CAD build for the part. Positions are in the model's coordinates, mm. Face numbers are marked on the shaded views. Coordinates: 2 decimals unless noted, no trailing zeros. Loops run counter-clockwise (first coordinate to the right, second up) from the corner with the lowest first, then second, coordinate; pieces in that order, holes last. Notation, with made-up numbers: (28.5, 8) -> (55.5, 8) arc R18 cw to (55.5, 25) -> close; hole circle Ø1 at (23, 52). An arc over 180 degrees is marked (long way). Write each question's results on one line, items separated by ' | '.
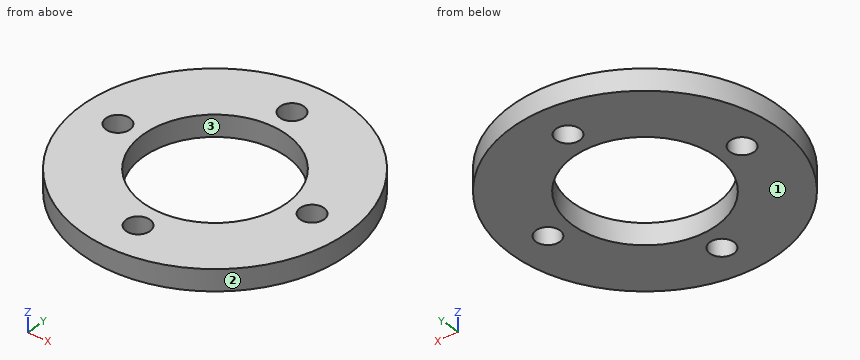
```python
from build123d import *

# Parameters (mm, degrees)
SKETCH1_R           = 25
SKETCH1_R_2         = 13.5
BOSS_EXTRUDE1_DEPTH = 4
SKETCH2_R           = 2.25
CUT_EXTRUDE1_DEPTH  = 5


with BuildPart() as part:
    # Sketch1 → Boss-Extrude1 (new body)
    with BuildSketch(Plane.XY):
        Circle(SKETCH1_R)
        Circle(SKETCH1_R_2, mode=Mode.SUBTRACT)
    extrude(amount=BOSS_EXTRUDE1_DEPTH)

    # Sketch2 → Cut-Extrude1 (cut, through all)
    with BuildSketch(Plane.XY.offset(4)):
        with Locations((0, 18)):
            Circle(SKETCH2_R)
        with Locations((18, 0)):
            Circle(SKETCH2_R)
        with Locations((0, -18)):
            Circle(SKETCH2_R)
        with Locations((-18, 0)):
            Circle(SKETCH2_R)
    extrude(amount=-CUT_EXTRUDE1_DEPTH, mode=Mode.SUBTRACT)


solid = part.part
```
Q1. Drop flat-ended pins along their axis: pin 1 (2 mm diameter, centred on x = -5.5, z = 2.5, fed in from -Y); pin 2 (4 mm diameter, centred on x = -18, y = 0, fed in from -Z); pin 3 (2 mm diameter, centred on y = 3.5, z = 2.5, fed in from +X); pin 4 (2 mm diameter, centred on x = 16, z = 2, fed in from +Y). Give the stop position or say it passes through.
Results are:
pin 1: y = -24.59 | pin 2: through | pin 3: x = 24.87 | pin 4: y = 20
Q2. Wall check: L1, parallel to X at y = -0.5, z = 3.3 (3 decimals); L2, parallel to X at y = 11.5, z = 0.6. Give the ranges that are in metal, low to high. Write a range as from..to.
Results are:
L1: -24.995..-20.194, -15.806..-13.491, 13.491..15.806, 20.194..24.995 | L2: -22.2..-7.07, 7.07..22.2
Q3. Cut at C-C on x = 7.5. Write the cut outline in (y, z), and give its area (3 significant figures).
Results are:
outline: (-23.85, 0) -> (-11.22, 0) -> (-11.22, 4) -> (-23.85, 4) -> close; (11.22, 0) -> (23.85, 0) -> (23.85, 4) -> (11.22, 4) -> close | area: 101 mm^2
Q4. Cut at A-A on x = 0. Write the cut outline in (y, z), and give its area (3 significant figures).
Results are:
outline: (-25, 0) -> (-20.25, 0) -> (-20.25, 4) -> (-25, 4) -> close; (-15.75, 0) -> (-13.5, 0) -> (-13.5, 4) -> (-15.75, 4) -> close; (13.5, 0) -> (15.75, 0) -> (15.75, 4) -> (13.5, 4) -> close; (20.25, 0) -> (25, 0) -> (25, 4) -> (20.25, 4) -> close | area: 56.0 mm^2
Q5. Pull direction X, two halves, no side cores. Call the marked faces 1, 2 and 3: +X half, -X half, draft (parallel to the pull), parting line (faces both ways), or undercut.
Results are:
face 1: draft | face 2: parting line | face 3: undercut
Q6. Cut at D-D on y = -18. Write the cut outline in (x, z), and give its area (3 significant figures).
Results are:
outline: (-17.35, 0) -> (-2.25, 0) -> (-2.25, 4) -> (-17.35, 4) -> close; (2.25, 0) -> (17.35, 0) -> (17.35, 4) -> (2.25, 4) -> close | area: 121 mm^2
